The model under review builds one solid part; all positions refer to its coordinate system, in mm. A direction names the side the tool comes from. Give positions to 0.01 mm unless a question says otherwise; leave off trailing zeros. Order: outer loops, then holes, each group sorted by start corner. A loop starts at its lowest first (then second) coordinate and runs counter-clockwise, first axis right, second up. Notation, with made-up numbers: (86, 81.5) - (116, 81.5) arc R21 cw to (116, 118.5) - close; hole circle Ø2 at (84, -25.75). An arc over 180 degrees is marked (long way). Write item = value, one per line. Start each with the question number.
1. We need section D-D, the plane y = 6. Give the boundary of the cut face in (x, z) (3 decimals).
2. For P1, Ø1.5, axis at x = -5.5, z = -7.5, coming from the -Y side; P2, Ø4.5, axis at y = -3.5, z = -26, coming from the +X side; P3, Ø8, axis at x = -5.5, z = 4, coming from the -Y side; P4, Ø5.5, axis at y = 0, z = -28.575, coming from the +X side, all flat-tipped, find the tip position at first contact; note any pin that passes through.
3. We need section B-B, the plane x = 0. Give the boundary of the cut face in (y, z) (3 decimals), and give its area (3 significant figures).
4. We need section A-A, the plane y = 0. Give the boundary of the cut face in (x, z) (3 decimals).
5. Wall thickness on probe 1 along Z at (x, y) = (-6.5, -2.25); probe 2 along X at (y, z) = (2.75, -22); probe 3 along X at (y, z) = (-8, -17.5): over which ranges is each line inside the solid? List them lowest first.
6. Machinability: for faces 5 (the flat face through (6.35, 0, -21)), 6 (the cylindrical face through (-9.11, -2.78, -2.75)), which of the approach directions +Z, -Z, +X, -X, +Y, -Y give a long, thin tool a straight path to every point of the face, cutting with its end or side? Answer none if there is none.
7. We need section C-C, the plane z = 10. Give the boundary of the cut face in (x, y) (3 decimals), and give its area (3 significant figures).
8. Mouldability with a two-part tool opening along Z and no side actions: class faces 1 (the cylindrical face through (-0.089, -1.932, -31.095)), 2 (the flat face through (-8, 0, -6.35)), 3 (the flat face through (-6.35, 0, -21)), 4 (the flat face through (0, 0, 13.208)) as pulls with the +Z half, pulls with the -Z half, needs draft (parallel to the pull), parting line crosses it, or undercut.
from build123d import *

# Parameters (mm, degrees)
SKETCH2_W           = 12.7
SKETCH2_H           = 60.004179461
CUT_EXTRUDE1_DEPTH  = 41.411152545
SKETCH3_R           = 3.175
CUT_EXTRUDE2_DEPTH  = 43.359783404
BOSS_EXTRUDE2_START = 13.208
SKETCH11_R          = 9.525
BOSS_EXTRUDE2_DEPTH = 13.208


with BuildPart() as part:
    # Sketch1 → Revolve1 (revolve)
    with BuildSketch(Plane(origin=(0, 0, 0), x_dir=(1, 0, 0), z_dir=(0, 1, 0)), mode=Mode.PRIVATE) as revolve1_sk:
        with BuildLine():
            Line((0, 0), (0, 28.575))
            Line((0, 28.575), (0, 38.1))
            ThreePointArc((0, 38.1), (6.735192091, 35.310192091), (9.525, 28.575))
            Line((9.525, 28.575), (9.525, 0))
            Line((9.525, 0), (0, 0))
        make_face()
    revolve(revolve1_sk.sketch.rotate(Axis((0, 0, -38.1), (0, 0, 1)), 180), axis=Axis((0, 0, -38.1), (0, 0, 1)))

    # Sketch2 → Cut-Extrude1 (cut, symmetric)
    with BuildSketch(Plane(origin=(0, 0, 0), x_dir=(1, 0, 0), z_dir=(0, 1, 0))):
        with Locations((-12.7, 36.35208973)):
            Rectangle(SKETCH2_W, SKETCH2_H)
    cut_extrude1 = extrude(amount=CUT_EXTRUDE1_DEPTH, both=True, mode=Mode.SUBTRACT)

    # Mirror1: Cut-Extrude1 across plane
    add(cut_extrude1.mirror(Plane(origin=(0, 0, 0), x_dir=(0, 0, 1), z_dir=(1, 0, 0))), mode=Mode.SUBTRACT)

    # Sketch3 → Cut-Extrude2 (cut, through all)
    with BuildSketch(Plane.ZY.offset(6.35)):
        with Locations((-28.575, 0)):
            Circle(SKETCH3_R)
    extrude(amount=-CUT_EXTRUDE2_DEPTH, mode=Mode.SUBTRACT)

    # Sketch11 → Boss-Extrude2 (add)
    with BuildSketch(Plane.XY.offset(BOSS_EXTRUDE2_START)):
        with Locations(Location((0, 0, 0), (0, 0, 131.810314896))):
            Circle(SKETCH11_R)
    extrude(amount=-BOSS_EXTRUDE2_DEPTH)


solid = part.part
Model answer:
q1.outline = (-7.398, -6.35) - (-6.35, -6.35) - (-6.35, -32.37) arc R7.398 ccw to (6.35, -32.37) - (6.35, -6.35) - (7.398, -6.35) - (7.398, 13.208) - (-7.398, 13.208) - close
q2.P1 = -8.26
q2.P2 = 6.35
q2.P3 = -9.41
q2.P4 = through
q3.outline = (-9.525, -28.575) arc R9.525 ccw to (9.525, -28.575) - (9.525, 13.208) - (-9.525, 13.208) - close; hole circle Ø6.35 at (0, -28.575)
q3.area = 907 mm2
q4.outline = (-9.525, -6.35) - (-6.35, -6.35) - (-6.35, -25.4) - (6.35, -25.4) - (6.35, -6.35) - (9.525, -6.35) - (9.525, 13.208) - (-9.525, 13.208) - close; (-6.35, -35.675) arc R9.525 ccw to (6.35, -35.675) - (6.35, -31.75) - (-6.35, -31.75) - close
q5.probe_1 = -6.35 to 13.21
q5.probe_2 = -6.35 to 6.35
q5.probe_3 = -5.17 to 5.17
q6.face_5 = -Z, +X, +Y, -Y
q6.face_6 = +Z, -Z
q7.outline = circle Ø19.05 at (0, 0)
q7.area = 285 mm2
q8.face_1 = undercut
q8.face_2 = pulls with the -Z half
q8.face_3 = needs draft
q8.face_4 = pulls with the +Z half
